Geometry: final body of the model. Coordinates: model frame, mm. A direction names the side the tool comes from. Round coordinates to 2 decimals unless told otherwise and drop trailing zeros. Loops run counter-clockwise (first coordinate to the right, second up) from the corner with the lowest first, then second, coordinate; pieces in that order, holes last. Notation, with made-up numbers: (48.5, 61) -> (105.5, 61) arc R12 ccw to (105.5, 67) -> close; hole circle Ø7 at (29, 46). An arc over 180 degrees is marked (long way). Answer in a Markdown table with one row per item.
```python
from build123d import *

# Parameters (mm, degrees)
SKETCH002_W      = 10.062535
SKETCH002_H      = 9.518799
EXTRUDE003_DEPTH = 80
SKETCH001_W      = 58
SKETCH001_H      = 125
SKETCH001_W_2    = 54
SKETCH001_H_2    = 121
EXTRUDE002_DEPTH = 6
SKETCH_W         = 70
SKETCH_H         = 140
EXTRUDE_DEPTH    = 5


with BuildPart() as legs:
    # Sketch002 → Extrude003 (new body)
    with BuildSketch(Plane.XY):
        with Locations((12.953979, 126.509788)):
            Rectangle(SKETCH002_W, SKETCH002_H)
        with Locations((56.843384, 126.509788)):
            Rectangle(SKETCH002_W, SKETCH002_H)
        with Locations((57.084308, 14.733897)):
            Rectangle(SKETCH002_W, SKETCH002_H)
        with Locations((13.107931, 14.733897)):
            Rectangle(SKETCH002_W, SKETCH002_H)
    extrude(amount=EXTRUDE003_DEPTH)


with BuildPart() as table_support:
    # Sketch001 → Extrude002 (new body)
    with BuildSketch(Plane.XY):
        with Locations((35, 70.5)):
            Rectangle(SKETCH001_W, SKETCH001_H)
        with Locations((35, 70.5)):
            Rectangle(SKETCH001_W_2, SKETCH001_H_2, mode=Mode.SUBTRACT)
    extrude(amount=EXTRUDE002_DEPTH)


with BuildPart() as table_support_1:
    # Extrude002 placement: moved
    add(table_support.part.moved(Location((0, 0, 6))))


with BuildPart() as fusion002:
    # Sketch → Extrude (new body)
    with BuildSketch(Plane.XY):
        with Locations((35, 70)):
            Rectangle(SKETCH_W, SKETCH_H)
    extrude(amount=EXTRUDE_DEPTH)

    # Fusion: union table_support
    add(table_support_1.part)

    # Fusion002: union legs
    add(legs.part)


solid = fusion002.part
```
Item 1: Section query B-B, the plane z = 22.5. Output: boundary loops of the cut face in (x, y), and give its area (3 significant figures).
Ans:
| item | result |
|---|---|
| outline | (7.92, 121.75) -> (17.99, 121.75) -> (17.99, 131.27) -> (7.92, 131.27) -> close; (8.08, 9.97) -> (18.14, 9.97) -> (18.14, 19.49) -> (8.08, 19.49) -> close; (51.81, 121.75) -> (61.87, 121.75) -> (61.87, 131.27) -> (51.81, 131.27) -> close; (52.05, 9.97) -> (62.12, 9.97) -> (62.12, 19.49) -> (52.05, 19.49) -> close |
| area | 383 mm2 |
Item 2: Section query A-A, the plane x = 27. Output: boundary loops of the cut face in (y, z).
Ans:
| item | result |
|---|---|
| outline | (0, 0) -> (140, 0) -> (140, 5) -> (0, 5) -> close; (8, 6) -> (10, 6) -> (10, 12) -> (8, 12) -> close; (131, 6) -> (133, 6) -> (133, 12) -> (131, 12) -> close |
Item 3: Section query C-C, the plane y = 56.5. Output: boundary loops of the cut face in (x, z).
Ans:
| item | result |
|---|---|
| outline | (0, 0) -> (70, 0) -> (70, 5) -> (0, 5) -> close; (6, 6) -> (8, 6) -> (8, 12) -> (6, 12) -> close; (62, 6) -> (64, 6) -> (64, 12) -> (62, 12) -> close |
Item 4: Section query D-D, the plane x = 58.5. Output: boundary loops of the cut face in (y, z).
Ans:
| item | result |
|---|---|
| outline | (0, 0) -> (140, 0) -> (140, 5) -> (131.27, 5) -> (131.27, 6) -> (133, 6) -> (133, 12) -> (131.27, 12) -> (131.27, 80) -> (121.75, 80) -> (121.75, 5) -> (19.49, 5) -> (19.49, 80) -> (9.97, 80) -> (9.97, 12) -> (8, 12) -> (8, 6) -> (9.97, 6) -> (9.97, 5) -> (0, 5) -> close |
Item 5: Ray query, L1, parallel to Y at x = 12, z = 77; L2, parallel to X at y = 98, z = 9.5; L3, parallel to Z at x = 47.5, y = 9.5. Return the intervals inside material, ascending.
Ans:
| item | result |
|---|---|
| L1 | 9.97 to 19.49, 121.75 to 131.27 |
| L2 | 6 to 8, 62 to 64 |
| L3 | 0 to 5, 6 to 12 |
Item 6: Mould query, pull axis X, two halves, no side actions, for faces 1 (the flat face through (51.812, 126, 42)), 2 (the flat face through (7.923, 126, 46)), 3 (the flat face through (35, 71, 0)), 4 (the flat face through (17.985, 126, 42)). Classes: released by +X, released by -X, zero draft, split by the parting line, or undercut.
Ans:
| item | result |
|---|---|
| face 1 | undercut |
| face 2 | released by -X |
| face 3 | zero draft |
| face 4 | undercut |
Item 7: Set-up query: faces 5 (the flat face through (13, 131.269, 46)), 6 (the flat face through (13, 9.974, 46)), 7 (the flat face through (35, 10, 9)). Return all of +Z, -Z, +X, -X, +Y, -Y with unobstructed straight access to the full face (end or side cutting, diameter ignored); none if empty.
Ans:
| item | result |
|---|---|
| face 5 | +Z, +X, -X, +Y |
| face 6 | +Z, +X, -X, -Y |
| face 7 | +Z |
Item 8: First-contact query: P1, Ø0.8, axis at x = 59, z = 5.5, coming from the +Y side; P2, Ø3, axis at x = 41.5, y = 93.5, coming from the -Z side; P3, Ø0.5, axis at x = 12, z = 5.5, coming from the -Y side; P4, Ø3, axis at y = 78, z = 8, coming from the +X side. Flat tips, straight axial feed; report the tip coordinate or a pass-through.
Ans:
| item | result |
|---|---|
| P1 | y = 131.27 |
| P2 | z = 0 |
| P3 | y = 9.97 |
| P4 | x = 64 |
